Autodesk Inventor part; units mm, degrees
ref_plane "YZ Plane" through (0, 0, 0) normal (1, 0, 0) x (0, 1, 0)
ref_plane "XZ Plane" through (0, 0, 0) normal (0, 1, 0) x (-1, 0, 0)
ref_plane "XY Plane" through (0, 0, 0) normal (0, 0, 1) x (1, 0, 0)
sketch "Sketch1" plane through (0, 0, 0) normal (0, 1, 0) x (-1, 0, 0)
  circle A0 centre (0, 0) radius 23
  circle A1 centre (0, 0) radius 19.25
  dimension "d2" = 46
  dimension "d3" = 38.5
extrude "Extrusion1" add sketch "Sketch1" along normal blind 18 draft 5
sketch "Sketch2" plane through (0, 0, 0) normal (0, -1, 0) x (1, 0, 0)
  circle A0 centre (0, 0) radius 19.25
  circle A1 centre (0, 0) radius 23
  circle A2 centre (0, 0) radius 24.5748
  circle A3 centre (0, 0) radius 17.6752
extrude "Extrusion2" cut sketch "Sketch2" against normal blind 15 contours A0 | A2 | A3
chamfer "Chamfer1" distance 1.3 angle 45 1 edges at (-23, 15, 0)
chamfer "Chamfer2" distance 1 angle 45 1 edges at (-19.25, 0, 0)
chamfer "Chamfer3" distance 0.5 angle 45 1 edges at (-23, 0, 0)
fillet "Fillet1" radius 2 2 edges at (17.6752, 18, 0) (24.5748, 18, 0)
chamfer "Chamfer4" distance 1.3 angle 45 1 edges at (-19.25, 15, 0)
properties part number "mesh-reseater"
Geometry check sheet. Reference: the model listing, model coordinates, mm. Round coordinates to 2 decimals unless told otherwise and drop trailing zeros. Order: outer loops, then holes, each group sorted by start corner. A loop starts at its lowest first (then second) coordinate and runs counter-clockwise, first axis right, second up. Notation, with made-up numbers: (8.25, 86.25) -> (25.25, 86.25) arc R24 ccw to (25.25, 119.25) -> close; hole circle Ø8 at (24, 30). An arc over 180 degrees is marked (long way). Use one line per item in the form item = value.
1. Mould release check, pull along X, two halves, no side actions. Record for faces 1 (the face through (17, 0, 12)), 2 (the face through (-15.28, 7.26, -11.71)), 3 (the face through (-2.994, 7.008, 22.804)): pulls with the +X half, pulls with the -X half, needs draft (parallel to the pull), parting line crosses it, or undercut.
Working result:
face_1 = needs draft
face_2 = undercut
face_3 = parting line crosses it
2. Scan lines: line 1 along Z through (x, y) = (0, 3.5); line 2 along X through (y, z) = (5.75, -0.5); line 3 along Z through (x, y) = (-11, 3). Record each from-to range of solid material in increasing order. Write a range as from..to.
Working result:
line_1 = -23..-19.25, 19.25..23
line_2 = -22.99..-19.24, 19.24..22.99
line_3 = -20.2..-15.8, 15.8..20.2
3. Go/stop test with flat-tipped pins: pin 1 (18 mm diameter, centred on x = 8, z = 2.5, fed in from -Y); pin 2 (14.5 mm diameter, centred on x = 8, z = 8.5, fed in from -Y); pin 3 (2 mm diameter, centred on y = 7.5, z = 0, fed in from -X); pin 4 (3 mm diameter, centred on x = 3.5, y = 7.5, fed in from +Z). Record where each tip stops, or that it passes through.
Working result:
pin_1 = through
pin_2 = 14.03
pin_3 = -23
pin_4 = 22.91
4. Cross-section at C-C, the plane y = 5.75. Enter the section's corners in (x, z), plus the area to 3 significant figures.
Working result:
outline = circle Ø46 at (0, 0); hole circle Ø38.5 at (0, 0)
area = 498 mm^2
5. Cross-section at D-D, the plane y = 17. Enter the section's corners in (x, z).
Working result:
outline = circle Ø48.25 at (0, 0); hole circle Ø36.25 at (0, 0)
